from build123d import *

# Parameters (mm, degrees)
BOSS_EXTRUDE1_DEPTH = 15
SKETCH2_R           = 10.6
CUT_EXTRUDE1_DEPTH  = 12
SKETCH3_R           = 6.5
CUT_EXTRUDE2_DEPTH  = 10
SKETCH4_R           = 2
CUT_EXTRUDE3_DEPTH  = 15


with BuildPart() as part:
    # Sketch1 → Boss-Extrude1 (new body)
    with BuildSketch(Plane.XY):
        with BuildLine():
            Line((-150, 160), (150, 160))
            ThreePointArc((150, 160), (157.071067812, 157.071067812), (160, 150))
            Line((160, 150), (160, -150))
            ThreePointArc((160, -150), (157.071067812, -157.071067812), (150, -160))
            Line((150, -160), (-150, -160))
            ThreePointArc((-150, -160), (-157.071067812, -157.071067812), (-160, -150))
            Line((-160, -150), (-160, 150))
            ThreePointArc((-160, 150), (-157.071067812, 157.071067812), (-150, 160))
        make_face()
    extrude(amount=BOSS_EXTRUDE1_DEPTH)

    # Sketch2 → Cut-Extrude1 (cut)
    with BuildSketch(Plane.XY.offset(15)):
        Circle(SKETCH2_R)
    extrude(amount=-CUT_EXTRUDE1_DEPTH, mode=Mode.SUBTRACT)

    # Sketch3 → Cut-Extrude2 (cut)
    with BuildSketch(Plane.XY.offset(3)):
        Circle(SKETCH3_R)
    extrude(amount=-CUT_EXTRUDE2_DEPTH, mode=Mode.SUBTRACT)

    # Sketch4 → Cut-Extrude3 (cut)
    with BuildSketch(Plane.XY.offset(15)):
        with Locations((0, 25)):
            Circle(SKETCH4_R)
        with Locations((25, 0)):
            Circle(SKETCH4_R)
        with Locations((0, -25)):
            Circle(SKETCH4_R)
        with Locations((-25, 0)):
            Circle(SKETCH4_R)
    extrude(amount=-CUT_EXTRUDE3_DEPTH, mode=Mode.SUBTRACT)


solid = part.part
Work out the finished part from the listing and answer in its coordinate system (mm). A direction names the side the tool comes from. Round coordinates to 2 decimals unless told otherwise and drop trailing zeros. One line per item, written item: value.
Q1. Straight lines are drawn through the part: probe 1 along Y at (x, z) = (0, 10.25); probe 2 along Y at (x, z) = (-25, 7.75); probe 3 along X at (y, z) = (1.5, 10.25). For each, find the intervals that lie inside material, in ascending order.
Check values:
probe 1: -160 to -27, -23 to -10.6, 10.6 to 23, 27 to 160
probe 2: -160 to -2, 2 to 160
probe 3: -160 to -26.32, -23.68 to -10.49, 10.49 to 23.68, 26.32 to 160
Q2. For faces 1 (the flat face through (160, 2, 7)), 2 (the cylindrical face through (9.79, -4.06, 9.08)), determine the directions among +Z, -Z, +X, -X, +Y, -Y from which every point of the face is accessible in a straight line to the end or side of a thin tool.
Check values:
face 1: +Z, -Z, +X, +Y, -Y
face 2: +Z
Q3. This flat-tipped pin is pushed along its axis until it touches: pin 1 Ø3.5 at (x, y) = (-25, 0) entering from +Z. Where does it stop, or does it pass through?
Check values:
pin 1: through
Q4. The mould has two halves that part along Y. Classify faces 3 (the flat face through (-33, 2, 15)), 4 (the cylindrical face through (157.15, -156.99, 7.4)), 5 (the cylindrical face through (-5.158, -3.955, 1.521)): +Y half, -Y half, draft (parallel to the pull), parting line (faces both ways), or undercut.
Check values:
face 3: draft
face 4: -Y half
face 5: undercut
